Input: part model. Units: mm. Frame: model coordinates. Give positions to 0.01 mm unless a question says otherwise; leave off trailing zeros. Write each loop counter-clockwise with the first axis right and the second up, starting at its lowest first coordinate (ties: lowest second). Pieces come first, ordered by that corner, then holes.
```python
from build123d import *

# Parameters (mm, degrees)
SKETCH1_W           = 67
SKETCH1_H           = 40
SKETCH1_R           = 13
SKETCH1_R_2         = 1.5
BOSS_EXTRUDE1_DEPTH = 3
CHAMFER1_SIZE       = 1


with BuildPart() as part:
    # Sketch1 → Boss-Extrude1 (new body)
    with BuildSketch(Plane.XY):
        with Locations((70.4, 127.33)):
            Rectangle(SKETCH1_W, SKETCH1_H)
        with Locations((54.9, 129.33)):
            Circle(SKETCH1_R, mode=Mode.SUBTRACT)
        with Locations((39.4, 129.33)):
            Circle(SKETCH1_R_2, mode=Mode.SUBTRACT)
        with Locations((54.9, 144.83)):
            Circle(SKETCH1_R_2, mode=Mode.SUBTRACT)
        with Locations((70.4, 129.33)):
            Circle(SKETCH1_R_2, mode=Mode.SUBTRACT)
        with Locations((54.9, 113.83)):
            Circle(SKETCH1_R_2, mode=Mode.SUBTRACT)
    extrude(amount=BOSS_EXTRUDE1_DEPTH)

    # Chamfer1
    chamfer1_edges = [part.edges().sort_by_distance(p)[0] for p in [
        (37.9, 129.33, 0),
        (68.9, 129.33, 0),
    ]]
    chamfer(chamfer1_edges, length=CHAMFER1_SIZE - 0.0001)  # a hair under: the kernel refuses the full size


solid = part.part
```
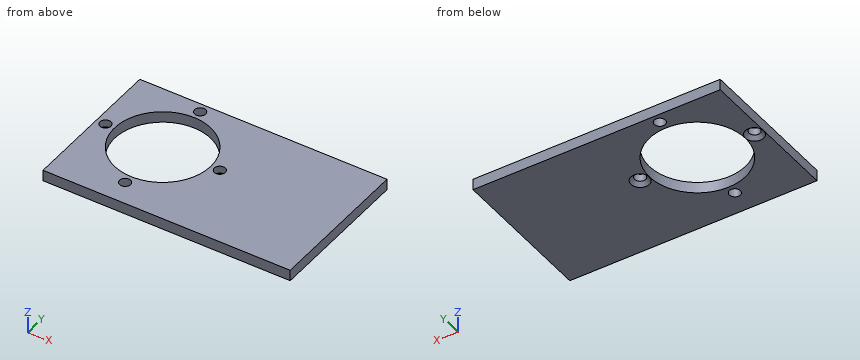
Item 1: Section A-A (y = 113.83). Return loops of the section in (x, z).
Item 2: Section D-D (x = 70.4). Return loops of the section in (y, z).
Item 3: Section B-B (x = 54.9). Return loops of the section in (y, z).
Item 4: Section C-C (z = 1.9). Return loops of the section in (x, y).
Item 5: Ray query, line 1 (Y direction, x = 54.9, z = 1.7); line 2 (X direction, y = 113.83, z = 1.4); line 3 (Y direction, x = 54.5, z = 2.4). Return the intervals inside material, ascending.
Item 6: Pin query (flat end, axial travel): pin 1 (2.5 mm diameter, centred on x = 70.4, y = 129.33, fed in from +Z). Return the tip coordinate at first contact, or that it passes through.
Solved:
1. outline: (36.9, 0) - (53.4, 0) - (53.4, 3) - (36.9, 3) - close; (56.4, 0) - (103.9, 0) - (103.9, 3) - (56.4, 3) - close
2. outline: (107.33, 0) - (126.83, 0) - (127.83, 1) - (127.83, 3) - (107.33, 3) - close; (130.83, 1) - (131.83, 0) - (147.33, 0) - (147.33, 3) - (130.83, 3) - close
3. outline: (107.33, 0) - (112.33, 0) - (112.33, 3) - (107.33, 3) - close; (115.33, 0) - (116.33, 0) - (116.33, 3) - (115.33, 3) - close; (142.33, 0) - (143.33, 0) - (143.33, 3) - (142.33, 3) - close; (146.33, 0) - (147.33, 0) - (147.33, 3) - (146.33, 3) - close
4. outline: (36.9, 107.33) - (103.9, 107.33) - (103.9, 147.33) - (36.9, 147.33) - close; hole circle Ø3 at (39.4, 129.33); hole circle Ø26 at (54.9, 129.33); hole circle Ø3 at (54.9, 113.83); hole circle Ø3 at (54.9, 144.83); hole circle Ø3 at (70.4, 129.33)
5. line 1: y = 107.33 to 112.33, 115.33 to 116.33, 142.33 to 143.33, 146.33 to 147.33
5. line 2: x = 36.9 to 53.4, 56.4 to 103.9
5. line 3: y = 107.33 to 112.38, 115.28 to 116.34, 142.32 to 143.38, 146.28 to 147.33
6. pin 1: passes through
